The listing builds one solid part. Answer for the finished solid, in the listing's coordinates (mm). A direction names the side the tool comes from. Give positions to 0.01 mm unless a question says otherwise; leave off trailing zeros. Order: outer loops, then holes, each group sorted by start corner. A loop starts at its lowest first (then second) coordinate and runs counter-clockwise, first axis right, second up. Notation, with made-up numbers: (-5.5, 35) - (31.5, 35) arc R13 cw to (31.5, 42) - close; hole circle Ø2 at (7.25, 54). An arc over 180 degrees is marked (long way). Use a Markdown table: item, result. Add a question column.
1) Find section D-D, the plane z = 0.7. State how many separate pieces and enclosed holes the cut face has, plus the area to 3 significant figures.
2) Find section A-A, the plane y = -0.5. Determine the outline of the cut face in (x, z), plus the area to 3 significant figures.
3) Straight lines are drawn through the part: line 1 (Z direction, x = 4, y = 4.5); line 2 (Y direction, x = 5, z = 0.75); line 3 (Y direction, x = 1, z = 0.8). For each, find the intervals that lie inside material, in ascending order.
4) For faces 1 (the face through (-6.35, -4.47, 0.92)), 2 (the face through (-6, 2, 0.45)), 3 (the face through (6.354, -4.456, 0.526)), determine the directions among +Z, -Z, +X, -X, +Y, -Y from which every point of the face is accessible in a straight line to the end or side of a thin tool.
5) Flat-ended cylindrical pins translate along their axes: pin 1 (0.7 mm diameter, centred on x = 4, y = -5.5, fed in from +Z); pin 2 (0.7 mm diameter, centred on y = -5, z = 0.5, fed in from +X). Find the tip coordinate at first contact, or state that the pin passes through.
6) The mould has two halves that part along Z. Classify faces 4 (the face through (-6, -1.05, 1)), 5 (the face through (1.27, -4.47, 0.92)), 6 (the face through (0, -2.55, 2)), 7 (the face through (-3.806, -4.456, 0.526)): released by +Z, released by -Z, zero draft, split by the parting line, or undercut.
7) Find section B-B, the plane x = -6.5. Determine the outline of the cut face in (y, z).
from build123d import *

# Parameters (mm, degrees)
SKETCH003_AS_DRAWN_W                      = 1.6
SKETCH003_AS_DRAWN_H                      = 1.6
EXTRUDE003_DEPTH                          = 7
EXTRUDE003_ONTO_SKETCH003_ROLL_ANGLE      = 90.0000000001
EXTRUDE003_ONTO_SKETCH003_PLACEMENT_ANGLE = 180
SKETCH002_W                               = 1.9
SKETCH002_H                               = 3.4
SKETCH002_W_2                             = 1.908066
SKETCH002_W_3                             = 1.08
SKETCH002_H_2                             = 3.401267
EXTRUDE002_DEPTH                          = 2.5
EXTRUDE001_DEPTH                          = 15.5
SKETCH_W                                  = 15.5
SKETCH_H                                  = 11.9
EXTRUDE_DEPTH                             = 2.5
FILLET_R                                  = 0.5


with BuildPart() as extrude003:
    # Sketch003 as drawn → Extrude003 (new)
    with BuildSketch(Plane.XY):
        with Locations((-1.27, 1.25)):
            Rectangle(SKETCH003_AS_DRAWN_W, SKETCH003_AS_DRAWN_H)
        with Locations((1.27, 1.25)):
            Rectangle(SKETCH003_AS_DRAWN_W, SKETCH003_AS_DRAWN_H)
        with Locations((3.81, 1.25)):
            Rectangle(SKETCH003_AS_DRAWN_W, SKETCH003_AS_DRAWN_H)
        with Locations((6.35, 1.25)):
            Rectangle(SKETCH003_AS_DRAWN_W, SKETCH003_AS_DRAWN_H)
        with Locations((-3.81, 1.25)):
            Rectangle(SKETCH003_AS_DRAWN_W, SKETCH003_AS_DRAWN_H)
        with Locations((-6.35, 1.25)):
            Rectangle(SKETCH003_AS_DRAWN_W, SKETCH003_AS_DRAWN_H)
    extrude(amount=-EXTRUDE003_DEPTH)


with BuildPart() as extrude003_1:
    # Extrude003 onto Sketch003 roll: moved
    add(extrude003.part.rotate(Axis((0, 0, 0), (1, 0, 0)), EXTRUDE003_ONTO_SKETCH003_ROLL_ANGLE))


with BuildPart() as extrude003_2:
    # Extrude003 onto Sketch003 placement: moved
    add(extrude003_1.part.moved(Location((0, 5.95, 0))).rotate(Axis((0, 5.95, 0), (0, 0, 1)), EXTRUDE003_ONTO_SKETCH003_PLACEMENT_ANGLE))


with BuildPart() as extrude002:
    # Sketch002 (on Face17 of Fillet) → Extrude002 (new body)
    with BuildSketch(Plane.XY.offset(2.5)):
        with Locations((-2.54, -4.25)):
            Rectangle(SKETCH002_W, SKETCH002_H)
        with Locations((0, -4.25)):
            Rectangle(SKETCH002_W, SKETCH002_H)
        with Locations((-5.084033, -4.25)):
            Rectangle(SKETCH002_W_2, SKETCH002_H)
        with Locations((5.08, -4.25)):
            Rectangle(SKETCH002_W, SKETCH002_H)
        with Locations((2.54, -4.25)):
            Rectangle(SKETCH002_W, SKETCH002_H)
        with Locations((-7.21, -4.2493665)):
            Rectangle(SKETCH002_W_3, SKETCH002_H_2)
        with Locations((7.21, -4.25)):
            Rectangle(SKETCH002_W_3, SKETCH002_H)
    extrude(amount=-EXTRUDE002_DEPTH)


with BuildPart() as extrude001:
    # Sketch001 (on Face2 of Extrude) → Extrude001 (new body)
    with BuildSketch(Plane.YZ.offset(7.75)):
        Polygon((-2.55, 2.5), (-5.95, 2.5), (-5.95, 0.4), (-5.1, 0.4), (-3.825, 1.45), (-2.55, 1.45), align=None)
        Polygon((-2.542972, 1.040645), (-3.825, 1.040645), (-5.1, 0), (-2.542972, 0), align=None)
    extrude(amount=-EXTRUDE001_DEPTH)


with BuildPart() as cut002:
    # Sketch → Extrude (new body)
    with BuildSketch(Plane.XY):
        Rectangle(SKETCH_W, SKETCH_H)
    extrude(amount=EXTRUDE_DEPTH)

    # Cut: cut Extrude001
    add(extrude001.part, mode=Mode.SUBTRACT)

    # Fillet
    fillet_edges = [cut002.edges().sort_by_distance(p)[0] for p in [
        (0, -5.1, 0),
        (0, -3.825, 1.040645),
        (0, -3.825, 1.45),
        (0, -5.1, 0.4),
    ]]
    fillet(fillet_edges, radius=FILLET_R)

    # Cut001: cut Extrude002
    add(extrude002.part, mode=Mode.SUBTRACT)

    # Cut002: cut Extrude003
    add(extrude003_2.part, mode=Mode.SUBTRACT)


solid = cut002.part
The answers:
| question | item | result |
|---|---|---|
| 1 | separate pieces | 7 |
| 1 | enclosed holes | 0 |
| 1 | area | 66.3 mm2 |
| 2 | outline | (-7.75, 0) - (7.75, 0) - (7.75, 2.5) - (-7.75, 2.5) - close; hole (-7.15, 0.45) - (-5.55, 0.45) - (-5.55, 2.05) - (-7.15, 2.05) - close; hole (-4.61, 0.45) - (-3.01, 0.45) - (-3.01, 2.05) - (-4.61, 2.05) - close; hole (-2.07, 0.45) - (-0.47, 0.45) - (-0.47, 2.05) - (-2.07, 2.05) - close; hole (0.47, 0.45) - (2.07, 0.45) - (2.07, 2.05) - (0.47, 2.05) - close; hole (3.01, 0.45) - (4.61, 0.45) - (4.61, 2.05) - (3.01, 2.05) - close; hole (5.55, 0.45) - (7.15, 0.45) - (7.15, 2.05) - (5.55, 2.05) - close |
| 2 | area | 23.4 mm2 |
| 3 | line 1 | 0 to 0.45, 2.05 to 2.5 |
| 3 | line 2 | -2.54 to 5.95 |
| 3 | line 3 | -4.61 to -4.12, -2.54 to -1.05 |
| 4 | face 1 | +Z, +X, -X, -Y |
| 4 | face 2 | +Y |
| 4 | face 3 | -Z, +X, -X |
| 5 | pin 1 | z = 0.42 |
| 5 | pin 2 | x = 6.67 |
| 6 | face 4 | undercut |
| 6 | face 5 | released by +Z |
| 6 | face 6 | zero draft |
| 6 | face 7 | released by -Z |
| 7 | outline | (-5.95, 0) - (-5.28, 0) arc R0.5 ccw to (-4.96, 0.11) - (-3.96, 0.93) arc R0.5 cw to (-3.65, 1.04) - (-2.54, 1.04) - (-2.54, 0) - (5.95, 0) - (5.95, 0.45) - (-1.05, 0.45) - (-1.05, 2.05) - (5.95, 2.05) - (5.95, 2.5) - (-2.55, 2.5) - (-2.55, 1.45) - (-3.65, 1.45) arc R0.5 ccw to (-3.96, 1.34) - (-4.96, 0.51) arc R0.5 cw to (-5.28, 0.4) - (-5.95, 0.4) - close |
